Work out the finished part from the listing and answer in its coordinate system (mm). Round coordinates to 2 decimals unless told otherwise and drop trailing zeros. Answer in a Markdown table with one row per item.
```python
from build123d import *

# Parameters (mm, degrees)
SKETCH1_W           = 577
SKETCH1_H           = 140
BOSS_EXTRUDE1_DEPTH = 6.35
SKETCH2_R           = 2
SKETCH2_R_2         = 1.75
SKETCH2_R_3         = 1.6
SKETCH2_R_4         = 1.5875
CUT_EXTRUDE1_DEPTH  = 297.93866791
SKETCH4_R           = 2.5
CUT_EXTRUDE2_DEPTH  = 297.93866791
CUT_EXTRUDE3_DEPTH  = 297.93866791


with BuildPart() as part:
    # Sketch1 → Boss-Extrude1 (new body)
    with BuildSketch(Plane.XY):
        Rectangle(SKETCH1_W, SKETCH1_H)
    extrude(amount=BOSS_EXTRUDE1_DEPTH)

    # Sketch2 → Cut-Extrude1 (cut, through all)
    with BuildSketch(Plane.XY.offset(6.35)):
        with Locations((75.619965266, 25)):
            Circle(SKETCH2_R)
        with Locations(Location((225.619965266, 25, 0), (0, 0, 180))):
            Circle(SKETCH2_R)
        with Locations((225.619965266, -25)):
            Circle(SKETCH2_R)
        with Locations(Location((75.619965266, -25, 0), (0, 0, 180))):
            Circle(SKETCH2_R)
        with Locations((16.996201668, 56)):
            Circle(SKETCH2_R)
        with Locations(Location((16.996201668, -56, 0), (0, 0, 180))):
            Circle(SKETCH2_R)
        with Locations((-25.003798332, 56)):
            Circle(SKETCH2_R)
        with Locations(Location((-25.003798332, -56, 0), (0, 0, 180))):
            Circle(SKETCH2_R)
        with Locations((-67.003798332, 56)):
            Circle(SKETCH2_R)
        with Locations(Location((-67.003798332, -56, 0), (0, 0, 180))):
            Circle(SKETCH2_R)
        with Locations((-109.003798332, 56)):
            Circle(SKETCH2_R)
        with Locations(Location((-109.003798332, -56, 0), (0, 0, 180))):
            Circle(SKETCH2_R)
        with Locations((-128.889819491, 51.768262599)):
            Circle(SKETCH2_R_2)
        with Locations(Location((-190.889819491, 51.768262599, 0), (0, 0, 180))):
            Circle(SKETCH2_R_2)
        with Locations(Location((-128.889819491, -27.231737401, 0), (0, 0, 180))):
            Circle(SKETCH2_R_2)
        with Locations((-190.889819491, -27.231737401)):
            Circle(SKETCH2_R_2)
        with Locations((268.371258164, 33)):
            Circle(SKETCH2_R_3)
        with Locations(Location((281.071258164, 33, 0), (0, 0, 180))):
            Circle(SKETCH2_R_3)
        with Locations((281.071258164, -33)):
            Circle(SKETCH2_R_3)
        with Locations(Location((268.371258164, -33, 0), (0, 0, 180))):
            Circle(SKETCH2_R_3)
        with Locations((-145.778767067, -54.079001217)):
            Circle(SKETCH2_R_4)
        with Locations((-175.828767067, -37.929001217)):
            Circle(SKETCH2_R_4)
        with Locations((178.481684403, 32.5)):
            Circle(SKETCH2_R)
        with Locations(Location((178.481684403, -32.5, 0), (0, 0, 180))):
            Circle(SKETCH2_R)
    extrude(amount=-CUT_EXTRUDE1_DEPTH, mode=Mode.SUBTRACT)

    # Sketch4 → Cut-Extrude2 (cut, through all)
    with BuildSketch(Plane.XY.offset(6.35)):
        with Locations((-273.5, 45)):
            Circle(SKETCH4_R)
        with Locations(Location((273.5, 45, 0), (0, 0, 180))):
            Circle(SKETCH4_R)
        with Locations((273.5, -45)):
            Circle(SKETCH4_R)
        with Locations(Location((-273.5, -45, 0), (0, 0, 180))):
            Circle(SKETCH4_R)
    extrude(amount=-CUT_EXTRUDE2_DEPTH, mode=Mode.SUBTRACT)

    # Sketch5 → Cut-Extrude3 (cut, through all)
    with BuildSketch(Plane.XY.offset(6.35)):
        with BuildLine():
            Line((-250.546207845, 56), (-210.546207845, 56))
            ThreePointArc((-210.546207845, 56), (-207.371207845, 52.825), (-210.546207845, 49.65))
            Line((-210.546207845, 49.65), (-250.546207845, 49.65))
            ThreePointArc((-250.546207845, 49.65), (-253.721207845, 52.825), (-250.546207845, 56))
        make_face()
        with BuildLine():
            Line((-250.546207845, 44.261111111), (-210.546207845, 44.261111111))
            ThreePointArc((-210.546207845, 44.261111111), (-207.371207845, 41.086111111), (-210.546207845, 37.911111111))
            Line((-210.546207845, 37.911111111), (-250.546207845, 37.911111111))
            ThreePointArc((-250.546207845, 37.911111111), (-253.721207845, 41.086111111), (-250.546207845, 44.261111111))
        make_face()
        with BuildLine():
            Line((-250.546207845, 32.522222222), (-210.546207845, 32.522222222))
            ThreePointArc((-210.546207845, 32.522222222), (-207.371207845, 29.347222222), (-210.546207845, 26.172222222))
            Line((-210.546207845, 26.172222222), (-250.546207845, 26.172222222))
            ThreePointArc((-250.546207845, 26.172222222), (-253.721207845, 29.347222222), (-250.546207845, 32.522222222))
        make_face()
        with BuildLine():
            Line((-250.546207845, 20.783333333), (-210.546207845, 20.783333333))
            ThreePointArc((-210.546207845, 20.783333333), (-207.371207845, 17.608333333), (-210.546207845, 14.433333333))
            Line((-210.546207845, 14.433333333), (-250.546207845, 14.433333333))
            ThreePointArc((-250.546207845, 14.433333333), (-253.721207845, 17.608333333), (-250.546207845, 20.783333333))
        make_face()
        with BuildLine():
            Line((-250.546207845, 9.044444444), (-210.546207845, 9.044444444))
            ThreePointArc((-210.546207845, 9.044444444), (-207.371207845, 5.869444444), (-210.546207845, 2.694444444))
            Line((-210.546207845, 2.694444444), (-250.546207845, 2.694444444))
            ThreePointArc((-250.546207845, 2.694444444), (-253.721207845, 5.869444444), (-250.546207845, 9.044444444))
        make_face()
        with BuildLine():
            Line((-250.546207845, -2.694444444), (-210.546207845, -2.694444444))
            ThreePointArc((-210.546207845, -2.694444444), (-207.371207845, -5.869444444), (-210.546207845, -9.044444444))
            Line((-210.546207845, -9.044444444), (-250.546207845, -9.044444444))
            ThreePointArc((-250.546207845, -9.044444444), (-253.721207845, -5.869444444), (-250.546207845, -2.694444444))
        make_face()
        with BuildLine():
            Line((-250.546207845, -14.433333333), (-210.546207845, -14.433333333))
            ThreePointArc((-210.546207845, -14.433333333), (-207.371207845, -17.608333333), (-210.546207845, -20.783333333))
            Line((-210.546207845, -20.783333333), (-250.546207845, -20.783333333))
            ThreePointArc((-250.546207845, -20.783333333), (-253.721207845, -17.608333333), (-250.546207845, -14.433333333))
        make_face()
        with BuildLine():
            Line((-250.546207845, -26.172222222), (-210.546207845, -26.172222222))
            ThreePointArc((-210.546207845, -26.172222222), (-207.371207845, -29.347222222), (-210.546207845, -32.522222222))
            Line((-210.546207845, -32.522222222), (-250.546207845, -32.522222222))
            ThreePointArc((-250.546207845, -32.522222222), (-253.721207845, -29.347222222), (-250.546207845, -26.172222222))
        make_face()
        with BuildLine():
            Line((-250.546207845, -37.911111111), (-210.546207845, -37.911111111))
            ThreePointArc((-210.546207845, -37.911111111), (-207.371207845, -41.086111111), (-210.546207845, -44.261111111))
            Line((-210.546207845, -44.261111111), (-250.546207845, -44.261111111))
            ThreePointArc((-250.546207845, -44.261111111), (-253.721207845, -41.086111111), (-250.546207845, -37.911111111))
        make_face()
        with BuildLine():
            Line((-250.546207845, -49.65), (-210.546207845, -49.65))
            ThreePointArc((-210.546207845, -49.65), (-207.371207845, -52.825), (-210.546207845, -56))
            Line((-210.546207845, -56), (-250.546207845, -56))
            ThreePointArc((-250.546207845, -56), (-253.721207845, -52.825), (-250.546207845, -49.65))
        make_face()
    extrude(amount=-CUT_EXTRUDE3_DEPTH, mode=Mode.SUBTRACT)


solid = part.part
```
1. The part is cut by section A-A (z = 3.75). Count the separate pieces of the cut face and the enclosed holes in it, plus the area to 3 significant figures.
Calculated:
| item | result |
|---|---|
| separate pieces | 1 |
| enclosed holes | 38 |
| area | 77,600 mm² |
2. Given pin 1 (4 mm diameter, centred on x = 143, y = -25, fed in from -Z); pin 2 (2.5 mm diameter, centred on x = 281.07, y = 33, fed in from -Z), each flat-ended and moving along its own axis, determine where each tip first touches the part or whether it passes through.
Calculated:
| item | result |
|---|---|
| pin 1 | stops at z = 0 |
| pin 2 | passes through |
3. Consider line 1 along Y through (x, z) = (-273.5, 5.25); line 2 along X through (y, z) = (-29.5, 0.5); line 3 along X through (y, z) = (24, 6). Determine where each line is inside the solid, lowest interval first. Write a range as from..to.
Calculated:
| item | result |
|---|---|
| line 1 | y = -70..-47.5, -42.5..42.5, 47.5..70 |
| line 2 | x = -288.5..-253.72, -207.37..288.5 |
| line 3 | x = -288.5..73.89, 77.35..223.89, 227.35..288.5 |
